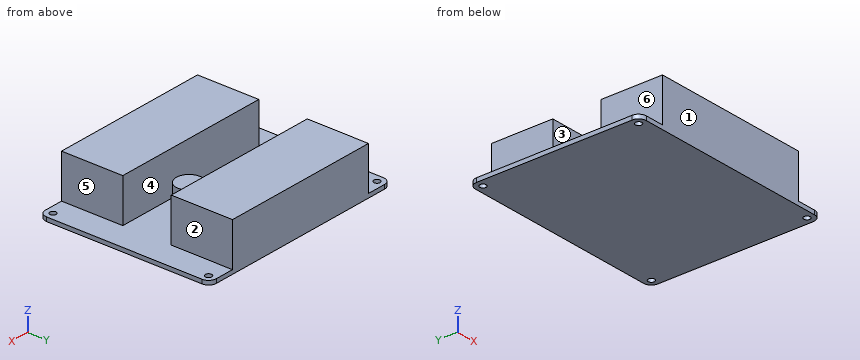
from build123d import *

# Parameters (mm, degrees)
PAD009_DEPTH    = 1.6
SKETCH027_R     = 1.25
POCKET010_DEPTH = 1.601
SKETCH028_R     = 5
PAD010_DEPTH    = 10
SKETCH029_W     = 63
SKETCH029_H     = 24
PAD011_DEPTH    = 17


with BuildPart() as part:
    # Sketch026 → Pad009 (new body)
    with BuildSketch(Plane.XY):
        with BuildLine():
            Line((39, 33.5), (-39, 33.5))
            ThreePointArc((-39, 33.5), (-41.12132, 32.62132), (-42, 30.5))
            Line((-42, 30.5), (-42, -30.5))
            ThreePointArc((-42, -30.5), (-41.12132, -32.62132), (-39, -33.5))
            Line((-39, -33.5), (39, -33.5))
            ThreePointArc((39, -33.5), (41.12132, -32.62132), (42, -30.5))
            Line((42, -30.5), (42, 30.5))
            ThreePointArc((42, 30.5), (41.12132, 32.62132), (39, 33.5))
        make_face()
    extrude(amount=PAD009_DEPTH)

    # Sketch027 (on Face10 of Pad009) → Pocket010 (cut, through all)
    with BuildSketch(Plane.XY.offset(1.6)):
        with Locations((-39, 30.5)):
            Circle(SKETCH027_R)
        with Locations((39, 30.5)):
            Circle(SKETCH027_R)
        with Locations((39, -30.5)):
            Circle(SKETCH027_R)
        with Locations((-39, -30.5)):
            Circle(SKETCH027_R)
    extrude(amount=-POCKET010_DEPTH, mode=Mode.SUBTRACT)

    # Sketch028 (on Face5 of Pocket010) → Pad010 (join)
    with BuildSketch(Plane.XY.offset(1.6)):
        with Locations((12, 0)):
            Circle(SKETCH028_R)
    extrude(amount=PAD010_DEPTH)

    # Sketch029 (on Face5 of Pad010) → Pad011 (join)
    with BuildSketch(Plane.XY.offset(1.6)):
        with Locations((0, 21.5)):
            Rectangle(SKETCH029_W, SKETCH029_H)
        with Locations((0, -21.5)):
            Rectangle(SKETCH029_W, SKETCH029_H)
    extrude(amount=PAD011_DEPTH)


solid = part.part
Can you work these out from the model? Positions are in its coordinate system, mm. Face numbers are marked on the shaded views. A direction names the side the tool comes from. Give positions to 0.01 mm unless a question says otherwise; leave off trailing zeros. Order: outer loops, then holes, each group sorted by start corner. A loop starts at its lowest first (then second) coordinate and runs counter-clockwise, first axis right, second up. Notation, with made-up numbers: M -20.5,13 L 31.5,13 A16 cw 31.5,26 Z; hole C 78,19.25 d5. An arc over 180 degrees is marked long. Use a Markdown table: item, result. Add a question column.
Item 1: Suppose I cut it at B-B (z = 17). List the corners of the cut face in (x, y) for me.
Item 2: Suppose I cut it at C-C (y = 0). List the corners of the cut face in (x, z) for me.
Item 3: Will these pins go through, and if not, where does the flat tip stop? pin 1 (8.5 mm diameter, centred on y = 20.5, z = 6.5, fed in from -X); pin 2 (2 mm diameter, centred on x = 39, y = 30.5, fed in from +Z); pin 3 (5 mm diameter, centred on y = -17.5, z = 9.5, fed in from +X); pin 4 (11 mm diameter, centred on x = 13.5, y = -0.5, fed in from +Z).
Item 4: Suppose I cut it at D-D (x = -6.5). List the corners of the cut face in (y, z) for me, then the cut area to 3 significant figures.
Item 5: Suppose I cut it at A-A (z = 3.75). List the corners of the cut face in (x, y) for me.
Item 6: We'd pull the mould along Y, two halves only. Please class the marked faces 1, 2 and 3: +Y half, -Y half, draft (parallel to the pull), parting line (faces both ways), or undercut.
Item 7: If I drill on L1, parallel to Y at x = 39, z = 1.3; L2, parallel to Y at x = -12.5, z = 8.5; L3, parallel to X at y = 30, z = 1, over which ranges is the centre line in solid material (lowest first)? Write a range as [from, to].
Item 8: For the marked faces 4, 5 and 6, which set-ups out of +Z, -Z, +X, -X, +Y, -Y let a thin tool reach every point of the face, with its end or its side?
Answer sheet:
| question | item | result |
|---|---|---|
| 1 | outline | M -31.5,-33.5 L 31.5,-33.5 L 31.5,-9.5 L -31.5,-9.5 Z; M -31.5,9.5 L 31.5,9.5 L 31.5,33.5 L -31.5,33.5 Z |
| 2 | outline | M -42,0 L 42,0 L 42,1.6 L 17,1.6 L 17,11.6 L 7,11.6 L 7,1.6 L -42,1.6 Z |
| 3 | pin 1 | stops at x = -31.5 |
| 3 | pin 2 | passes through |
| 3 | pin 3 | stops at x = 31.5 |
| 3 | pin 4 | stops at z = 11.6 |
| 4 | outline | M -33.5,0 L 33.5,0 L 33.5,18.6 L 9.5,18.6 L 9.5,1.6 L -9.5,1.6 L -9.5,18.6 L -33.5,18.6 Z |
| 4 | area | 923 mm² |
| 5 | outline | M -31.5,-33.5 L 31.5,-33.5 L 31.5,-9.5 L -31.5,-9.5 Z; M -31.5,9.5 L 31.5,9.5 L 31.5,33.5 L -31.5,33.5 Z; C 12,0 d10 |
| 6 | face 1 | -Y half |
| 6 | face 2 | draft |
| 6 | face 3 | undercut |
| 7 | L1 | y = [-33.5, -31.75], [-29.25, 29.25], [31.75, 33.5] |
| 7 | L2 | y = [-33.5, -9.5], [9.5, 33.5] |
| 7 | L3 | x = [-42, -40.15], [-37.85, 37.85], [40.15, 42] |
| 8 | face 4 | +Z, +X, -X |
| 8 | face 5 | +Z, +X, +Y, -Y |
| 8 | face 6 | +Z, -X, +Y, -Y |
